Could you check a few things on this drawing? It's one solid part, dimensions in mm from its lowest x, y, z. A direction names the side the tool comes from. Give positions to 0.01 mm unless a question says otherwise; leave off trailing zeros. Return JSON: item names as keys, results as strings. Group by question number.
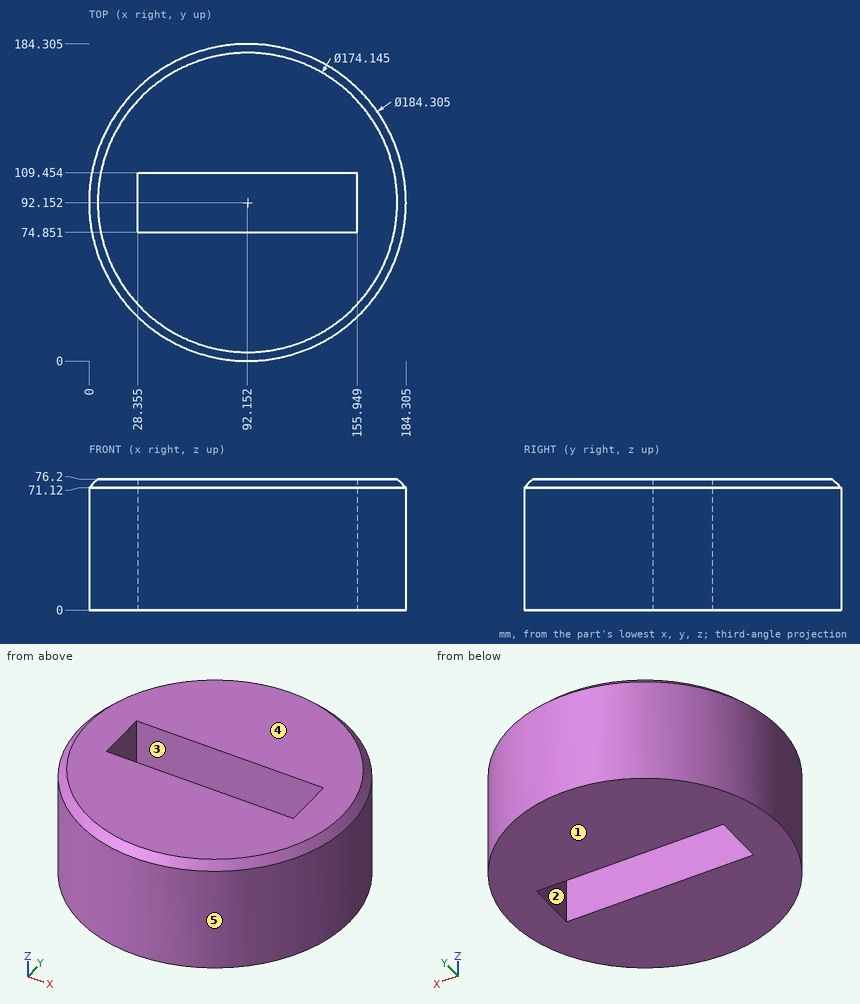
1. For pin 1 (8 mm diameter, centred on x = 19.5, z = 33, fed in from -Y); pin 2 (3 mm diameter, centred on x = 36, z = 46.5, fed in from -Y) (1 decimal); pin 3 (2 mm diameter, centred on x = 59.5, z = 50, fed in from -Y), each with a flat end and sliding along its axis, tell me the tip position at first contact or that it passes through.
2. If we mould it in two halves opening along Y, with no side actions, what happens to the marked faces 3, 4 and 5? For each: pulls with the +Y half, pulls with the -Y half, needs draft (parallel to the pull), parting line crosses it, or undercut.
3. I need wall thicknesses on L1, parallel to Y at x = 91, z = 39; L2, parallel to Y at x = 96, z = 52 (1 decimal); L3, parallel to Y at x = 27, z = 47.5 (1 decimal). Which ranges of each line are inside material? Lowest first, please. Write a range as from..to.
4. Which directions (+Z, -Z, +X, -X, +Y, -Y) give clear straight access to the entire face, cutting with the end or side of a thin tool? Please do the marked faces 1 and 2.
Values:
{
 "1": {"pin 1": "stops at y = 30.68", "pin 2": "stops at y = 18", "pin 3": "stops at y = 5.61"},
 "2": {"face 3": "undercut", "face 4": "needs draft", "face 5": "parting line crosses it"},
 "3": {"L1": "y = 0.01..74.85, 109.45..184.3", "L2": "y = 0.1..74.9, 109.5..184.2", "L3": "y = 27..157.3"},
 "4": {"face 1": "-Z, +X, -X, +Y, -Y", "face 2": "+Z, -Z"}
}
